The figure shows three views and two pictorial views of one solid part (mm, origin at its lowest corner). Answer the questions. A direction names the side the tool comes from. Give positions to 0.01 mm unless a question says otherwise; leave off trailing zeros. Order: outer loops, then holes, each group sorted by start corner. A loop starts at its lowest first (then second) coordinate and runs counter-clockwise, first axis right, second up. Notation, with made-up numbers: (46.5, -31.5) - (82.5, -31.5) arc R9 cw to (82.5, -14.5) - close; hole circle Ø11 at (39.25, -6.5). An arc over 180 degrees is marked (long way). Answer as a JSON object with one key per item and string values. Group by question number.
Q1. A cutting plane is placed at D-D, the plane z = 17. Give the vertices of the cut face in (x, y).
Q2. A cutting plane is placed at B-B, the plane y = 19.5. Give the vertices of the cut face in (x, z).
Q3. A cutting plane is placed at C-C, the plane x = 16.75. Give the vertices of the cut face in (y, z).
Q4. A cutting plane is placed at A-A, the plane z = 10. Give the vertices of the cut face in (x, y).
Q5. For the marked faces 5 and 6, determine the directions among +Z, -Z, +X, -X, +Y, -Y from which every point of the face is accessible in a straight line to the end or side of a thin tool.
Q6. Consider line 1 (Z direction, x = 18.7, y = 10); line 2 (X direction, y = 7.5, z = 13); line 3 (Z direction, x = 0.9, y = 30). Determine where each line is inside the solid, lowest interval first.
Q7. Given pin 1 (17 mm diameter, centred on y = 10.5, z = 12, fed in from -X); pin 2 (12 mm diameter, centred on x = 12, z = 18.5, fed in from +Y); pin 3 (6 mm diameter, centred on x = 11.5, y = 16.5, fed in from +Z); pin 4 (2 mm diameter, centred on y = 10, z = 10, fed in from +X), each flat-ended and moving along its own axis, determine where each tip first touches the part or whether it passes through.
Q8. The mould has two halves that part along Z. Classify the marked faces 1, 2, 3 and 4: released by +Z, released by -Z, zero draft, split by the parting line, or undercut.
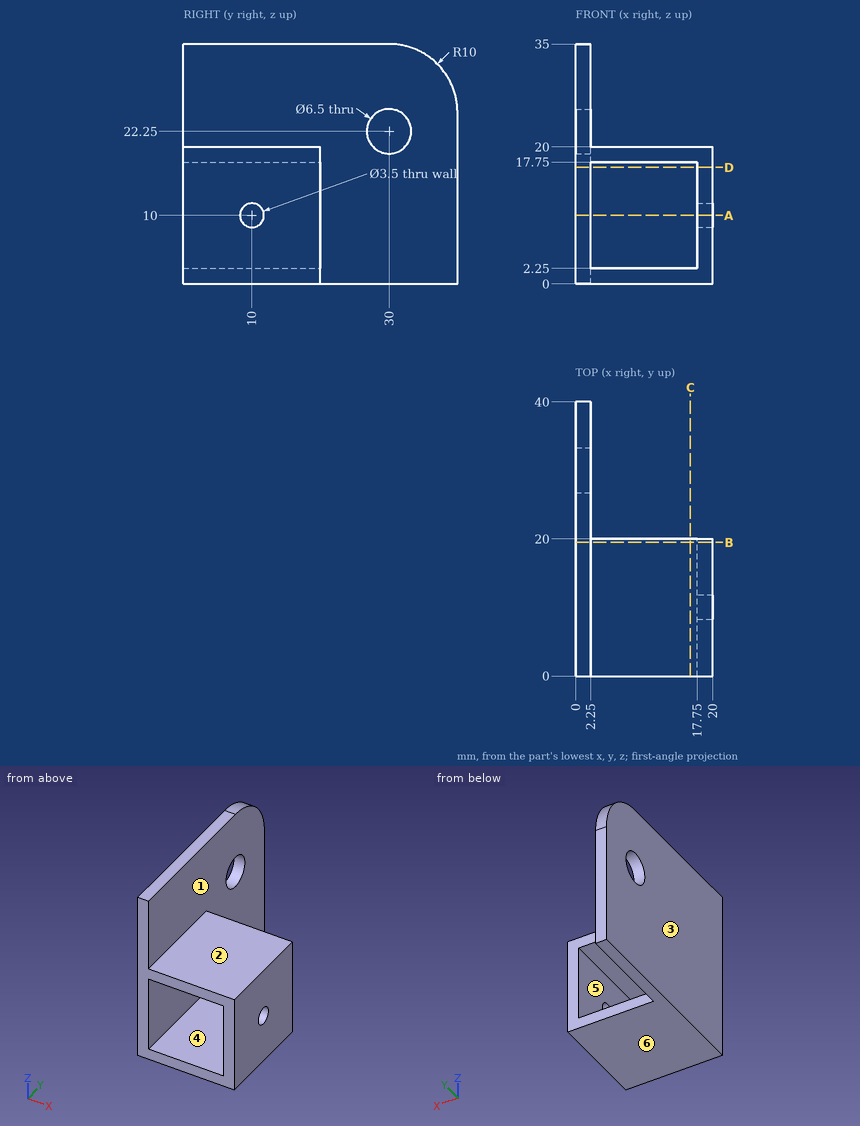
Reply:
{
 "1": {"outline": "(0, 0) - (2.25, 0) - (2.25, 40) - (0, 40) - close; (17.75, 0) - (20, 0) - (20, 20) - (17.75, 20) - close"},
 "2": {"outline": "(0, 0) - (20, 0) - (20, 20) - (2.25, 20) - (2.25, 35) - (0, 35) - close; hole (2.25, 2.25) - (17.75, 2.25) - (17.75, 17.75) - (2.25, 17.75) - close"},
 "3": {"outline": "(0, 0) - (20, 0) - (20, 2.25) - (0, 2.25) - close; (0, 17.75) - (20, 17.75) - (20, 20) - (0, 20) - close"},
 "4": {"outline": "(0, 0) - (2.25, 0) - (2.25, 40) - (0, 40) - close; (17.75, 0) - (20, 0) - (20, 8.25) - (17.75, 8.25) - close; (17.75, 11.75) - (20, 11.75) - (20, 20) - (17.75, 20) - close"},
 "5": {"face 5": "+Y, -Y", "face 6": "-Z, +X, -X, +Y, -Y"},
 "6": {"line 1": "z = 0 to 8.25, 11.75 to 20", "line 2": "x = 0 to 2.25, 17.75 to 20", "line 3": "z = 0 to 19, 25.5 to 35"},
 "7": {"pin 1": "stops at x = 0", "pin 2": "stops at y = 20", "pin 3": "stops at z = 20", "pin 4": "stops at x = 2.25"},
 "8": {"face 1": "undercut", "face 2": "released by +Z", "face 3": "zero draft", "face 4": "undercut"}
}
